Verification items for the finished model (mm, model axes). A direction names the side the tool comes from. Coordinates: 2 decimals unless noted, no trailing zeros. Loops run counter-clockwise (first coordinate to the right, second up) from the corner with the lowest first, then second, coordinate; pieces in that order, holes last. Notation, with made-up numbers: (23, 88.25) - (79, 88.25) arc R10 cw to (79, 95.25) - close; hole circle Ø1 at (63.25, 6). An arc over 180 degrees is marked (long way). One line per item, written item: value. Start each with the question number.
(1) Section check B-B (x = 137). Record the boundary of the cut face in (y, z), plus the area to 3 significant figures.
(2) Draft check along Z on faces 1 (the face through (145, 56, 21)), 2 (the face through (144, 57, 24)), 3 (the face through (145, 113, 22)), 4 (the face through (89, 91, 0)). Enter one of: +Z half, -Z half, draft (parallel to the pull), parting line (faces both ways), or undercut.
(3) Section check C-C (y = 134). Record the boundary of the cut face in (x, z), plus the area to 3 significant figures.
(4) Thickness scan on probe 1 along Y at (x, z) = (80, 2); probe 2 along Y at (x, z) = (159.5, 22.05); probe 3 along X at (y, z) = (74, 17.5). Record the ranges inside material, lowest first. Write a range as [from, to].
(5) Section check D-D (y = 96). Record the boundary of the cut face in (x, z).
(6) Section check A-A (x = 170). Record the boundary of the cut face in (y, z), plus the area to 3 significant figures.
(7) Gauge pin test, flat ends, axial feed: P1, Ø5.5, axis at x = 15, y = 40, coming from the -Z side; P2, Ø1, axis at y = 100, z = 15, coming from the -X side; P3, Ø1, axis at x = 128, z = 12, coming from the +Y side. Record the tip position at first contact, or that the pin passes through.
(8) Set-up check for faces 5 (the face through (158.026, 106.352, 1.521)), 6 (the face through (109, 56, 13)), 7 (the face through (89, 91, 3)): record each of +Z, -Z, +X, -X, +Y, -Y from which the full face is reachable in a straight line by a thin tool's end or side.
```python
from build123d import *

# Parameters (mm, degrees)
SKETCH_W        = 180
SKETCH_H        = 180
SKETCH_R        = 2.5
SKETCH_W_2      = 50
SKETCH_H_2      = 40
PAD_DEPTH       = 3
PAD001_DEPTH    = 21
SKETCH002_W     = 113
SKETCH002_H     = 3
PAD002_DEPTH    = 71
SKETCH003_R     = 2
POCKET_DEPTH    = 100
SKETCH004_R     = 1.75
POCKET001_DEPTH = 5
SKETCH005_R     = 1.75
POCKET002_DEPTH = 5


with BuildPart() as part:
    # Sketch → Pad (new body)
    with BuildSketch(Plane.XY):
        with Locations((90, 90)):
            Rectangle(SKETCH_W, SKETCH_H)
        with Locations((90, 25)):
            Circle(SKETCH_R, mode=Mode.SUBTRACT)
        with Locations((10, 170)):
            Circle(SKETCH_R, mode=Mode.SUBTRACT)
        with Locations((170, 170)):
            Circle(SKETCH_R, mode=Mode.SUBTRACT)
        with Locations((135, 140)):
            Rectangle(SKETCH_W_2, SKETCH_H_2, mode=Mode.SUBTRACT)
    extrude(amount=PAD_DEPTH)

    # Sketch001 (on Face13 of Pad) → Pad001 (join)
    with BuildSketch(Plane.XY.offset(3)):
        Polygon((180, 0), (180, 113), (177, 113), (177, 3), (157, 3), (157, 0), align=None)
        Polygon((112, 113), (112, 3), (132, 3), (132, 0), (109, 0), (109, 113), align=None)
    extrude(amount=PAD001_DEPTH)

    # Sketch002 (on Face9 of Pad001) → Pad002 (join)
    with BuildSketch(Plane.YZ.offset(180)):
        with Locations((56.5, 22.5)):
            Rectangle(SKETCH002_W, SKETCH002_H)
    extrude(amount=-PAD002_DEPTH)

    # Sketch003 (on Face37 of Pad002) → Pocket (cut)
    with BuildSketch(Plane.XY.offset(24)):
        with Locations((129.5, 105)):
            Circle(SKETCH003_R)
        with Locations((144.5, 105)):
            Circle(SKETCH003_R)
        with Locations((159.5, 105)):
            Circle(SKETCH003_R)
    extrude(amount=-POCKET_DEPTH, mode=Mode.SUBTRACT)

    # Sketch004 (on Face5 of Pocket) → Pocket001 (cut)
    with BuildSketch(Plane.XY.offset(3)):
        with Locations((75, 170)):
            Circle(SKETCH004_R)
        with Locations((105, 170)):
            Circle(SKETCH004_R)
        with Locations((75, 140)):
            Circle(SKETCH004_R)
        with Locations((105, 140)):
            Circle(SKETCH004_R)
    extrude(amount=-POCKET001_DEPTH, mode=Mode.SUBTRACT)

    # Sketch005 (on Face5 of Pocket001) → Pocket002 (cut)
    with BuildSketch(Plane.XY.offset(3)):
        with Locations((15, 15)):
            Circle(SKETCH005_R)
        with Locations((15, 40)):
            Circle(SKETCH005_R)
        with Locations((40, 40)):
            Circle(SKETCH005_R)
        with Locations((40, 15)):
            Circle(SKETCH005_R)
        with Locations((80, 40)):
            Circle(SKETCH005_R)
        with Locations((80, 15)):
            Circle(SKETCH005_R)
    extrude(amount=-POCKET002_DEPTH, mode=Mode.SUBTRACT)


solid = part.part
```
Responses:
1. outline: (0, 0) - (120, 0) - (120, 3) - (0, 3) - close; (0, 21) - (113, 21) - (113, 24) - (0, 24) - close; (160, 0) - (180, 0) - (180, 3) - (160, 3) - close
1. area: 759 mm²
2. face 1: undercut
2. face 2: +Z half
2. face 3: draft
2. face 4: -Z half
3. outline: (0, 0) - (110, 0) - (110, 3) - (0, 3) - close; (160, 0) - (180, 0) - (180, 3) - (160, 3) - close
3. area: 390 mm²
4. probe 1: y = [0, 13.25], [16.75, 38.25], [41.75, 180]
4. probe 2: y = [0, 103], [107, 113]
4. probe 3: x = [109, 112], [177, 180]
5. outline: (0, 0) - (180, 0) - (180, 24) - (109, 24) - (109, 3) - (0, 3) - close; hole (112, 3) - (177, 3) - (177, 21) - (112, 21) - close
6. outline: (0, 0) - (167.5, 0) - (167.5, 3) - (3, 3) - (3, 21) - (113, 21) - (113, 24) - (0, 24) - close; (172.5, 0) - (180, 0) - (180, 3) - (172.5, 3) - close
6. area: 918 mm²
7. P1: stops at z = 0
7. P2: stops at x = 109
7. P3: stops at y = 3
8. face 5: +Z, -Z
8. face 6: +Z, -X, +Y, -Y
8. face 7: +Y
